For this review, take the finished solid that the model builds, in its own axes (mm). A direction names the side the tool comes from. Coordinates: 2 decimals unless noted, no trailing zeros. Write each loop counter-clockwise with the first axis right and the second up, starting at its lowest first coordinate (ties: lowest second). Pieces come first, ordered by that corner, then holes.
```python
from build123d import *

# Parameters (mm, degrees)
BOSS_EXTRUDE1_DEPTH = 370
SKETCH2_R           = 4.05
CUT_EXTRUDE1_DEPTH  = 26
CUT_EXTRUDE2_REACH  = 27
CUT_EXTRUDE3_REACH  = 27
SKETCH4_R           = 6


with BuildPart() as part:
    # Sketch1 → Boss-Extrude1 (new body)
    with BuildSketch(Plane.XY):
        with BuildLine():
            Line((2, 0), (23, 0))
            ThreePointArc((23, 0), (24.414213562, 0.585786438), (25, 2))
            Line((25, 2), (25, 23))
            ThreePointArc((25, 23), (24.414213562, 24.414213562), (23, 25))
            Line((23, 25), (2, 25))
            ThreePointArc((2, 25), (0.585786438, 24.414213562), (0, 23))
            Line((0, 23), (0, 2))
            ThreePointArc((0, 2), (0.585786438, 0.585786438), (2, 0))
        make_face()
        with BuildLine():
            Line((2, 1.25), (23, 1.25))
            ThreePointArc((23, 1.25), (23.530330086, 1.469669914), (23.75, 2))
            Line((23.75, 2), (23.75, 23))
            ThreePointArc((23.75, 23), (23.530330086, 23.530330086), (23, 23.75))
            Line((23, 23.75), (2, 23.75))
            ThreePointArc((2, 23.75), (1.469669914, 23.530330086), (1.25, 23))
            Line((1.25, 23), (1.25, 2))
            ThreePointArc((1.25, 2), (1.469669914, 1.469669914), (2, 1.25))
        make_face(mode=Mode.SUBTRACT)
    extrude(amount=BOSS_EXTRUDE1_DEPTH)

    # Sketch2 → Cut-Extrude1 (cut, through all)
    with BuildSketch(Plane(origin=(0, 25, 0), x_dir=(1, 0, 0), z_dir=(0, 1, 0))):
        with Locations((12.5, -293)):
            Circle(SKETCH2_R)
        with BuildLine():
            Line((8.45, -353), (8.45, -370))
            Line((8.45, -370), (16.55, -370))
            Line((16.55, -370), (16.55, -353))
            ThreePointArc((16.55, -353), (12.5, -348.95), (8.45, -353))
        make_face()
    extrude(amount=-CUT_EXTRUDE1_DEPTH, mode=Mode.SUBTRACT)

    # Sketch3 → Cut-Extrude2 (cut, up to next)
    with BuildSketch(Plane(origin=(0, 25, 0), x_dir=(1, 0, 0), z_dir=(0, 1, 0)), mode=Mode.PRIVATE) as cut_extrude2_sk1:
        with BuildLine():
            Line((17.05, -38), (17.05, -70))
            ThreePointArc((17.05, -70), (12.5, -74.55), (7.95, -70))
            Line((7.95, -70), (7.95, -38))
            ThreePointArc((7.95, -38), (12.5, -33.45), (17.05, -38))
        make_face()
    cut_extrude2_tool1 = extrude(cut_extrude2_sk1.sketch, amount=-CUT_EXTRUDE2_REACH, mode=Mode.PRIVATE) & part.part
    add(cut_extrude2_tool1.solids().sort_by_distance((12.5, 25, 54))[0], mode=Mode.SUBTRACT)

    # Sketch4 → Cut-Extrude3 (cut, up to next)
    with BuildSketch(Plane.XZ, mode=Mode.PRIVATE) as cut_extrude3_sk1:
        with Locations((12.5, 53)):
            Circle(SKETCH4_R)
    cut_extrude3_tool1 = extrude(cut_extrude3_sk1.sketch, amount=-CUT_EXTRUDE3_REACH, mode=Mode.PRIVATE) & part.part
    add(cut_extrude3_tool1.solids().sort_by_distance((12.5, 0, 53))[0], mode=Mode.SUBTRACT)
    # Sketch4 → Cut-Extrude3 (cut, up to next)
    with BuildSketch(Plane.XZ, mode=Mode.PRIVATE) as cut_extrude3_sk2:
        with BuildLine():
            Line((7.95, 0), (7.95, 17))
            ThreePointArc((7.95, 17), (12.5, 21.55), (17.05, 17))
            Line((17.05, 17), (17.05, 0))
            Line((17.05, 0), (7.95, 0))
        make_face()
    cut_extrude3_tool2 = extrude(cut_extrude3_sk2.sketch, amount=-CUT_EXTRUDE3_REACH, mode=Mode.PRIVATE) & part.part
    add(cut_extrude3_tool2.solids().sort_by_distance((12.5, 0, 10.311845))[0], mode=Mode.SUBTRACT)


solid = part.part
```
Q1. Add section D-D (z = 293). State the section outline as (x, y) points, then the cut area to 3 significant figures.
Ans:
outline: (0, 2) arc R2 ccw to (2, 0) - (8.45, 0) - (8.45, 1.25) - (2, 1.25) arc R0.75 cw to (1.25, 2) - (1.25, 23) arc R0.75 cw to (2, 23.75) - (8.45, 23.75) - (8.45, 25) - (2, 25) arc R2 ccw to (0, 23) - close; (16.55, 0) - (23, 0) arc R2 ccw to (25, 2) - (25, 23) arc R2 ccw to (23, 25) - (16.55, 25) - (16.55, 23.75) - (23, 23.75) arc R0.75 cw to (23.75, 23) - (23.75, 2) arc R0.75 cw to (23, 1.25) - (16.55, 1.25) - close
area: 95.5 mm2
Q2. Add section C-C (x = 12.5). State the section outline as (y, z) points, then the cut area to 3 significant figures.
Ans:
outline: (0, 21.55) - (1.25, 21.55) - (1.25, 47) - (0, 47) - close; (0, 59) - (1.25, 59) - (1.25, 288.95) - (0, 288.95) - close; (0, 297.05) - (1.25, 297.05) - (1.25, 348.95) - (0, 348.95) - close; (23.75, 0) - (25, 0) - (25, 33.45) - (23.75, 33.45) - close; (23.75, 74.55) - (25, 74.55) - (25, 288.95) - (23.75, 288.95) - close; (23.75, 297.05) - (25, 297.05) - (25, 348.95) - (23.75, 348.95) - close
area: 759 mm2
Q3. Clearance check with flat-ended pins moving along their axes: pin 1 Ø0.6 at (y, z) = (1, 361.5) entering from -X; pin 2 Ø1.4 at (y, z) = (24, 50) entering from +X; pin 3 Ø1.4 at (y, z) = (0.5, 7) entering from -X; pin 4 Ø8 at (x, y) = (15, 19) entering from -Z. State where each tip first meets the part, or that it passes through.
Ans:
pin 1: stops at x = 0.13
pin 2: stops at x = 24.98
pin 3: stops at x = 0.17
pin 4: passes through
Q4. Tool access review of faces 1 (the flat face through (24, 13, 370)), 2 (the cylindrical face through (18.04, 0.62, 50.7)), 3 (the flat face through (23.75, 12, 182)): name each direction out of +Z, -Z, +X, -X, +Y, -Y from which nothing blocks a thin tool from reaching the whole face with its end or side.
Ans:
face 1: +Z, +X, -X, +Y, -Y
face 2: -Y
face 3: +Z, -Z
Q5. Add section A-A (y = 11.25). State the section outline as (x, z) points.
Ans:
outline: (0, 0) - (1.25, 0) - (1.25, 370) - (0, 370) - close; (23.75, 0) - (25, 0) - (25, 370) - (23.75, 370) - close
Q6. For probe 1 along Z at (x, y) = (12.5, 24.15); probe 2 along Z at (x, y) = (12.5, 0.5); probe 3 along Y at (x, z) = (19.5, 221.5), list the stretches that pass through material, from the lowest coordinate up.
Ans:
probe 1: z = 0 to 33.45, 74.55 to 288.95, 297.05 to 348.95
probe 2: z = 21.55 to 47, 59 to 288.95, 297.05 to 348.95
probe 3: y = 0 to 1.25, 23.75 to 25
Q7. Draft analysis for pull direction Y (two halves, no side actions). For faces 4 (the flat face through (12, 1.25, 182)), 5 (the flat face through (25, 12, 182)), 6 (the flat face through (1.25, 13, 182)), 7 (the flat face through (13, 25, 182)), state which applies: +Y half, -Y half, draft (parallel to the pull), parting line (faces both ways), or undercut.
Ans:
face 4: undercut
face 5: draft
face 6: undercut
face 7: +Y half
Q8. Add section B-B (z = 199.5). State the section outline as (x, y) points, then the cut area to 3 significant figures.
Ans:
outline: (0, 2) arc R2 ccw to (2, 0) - (23, 0) arc R2 ccw to (25, 2) - (25, 23) arc R2 ccw to (23, 25) - (2, 25) arc R2 ccw to (0, 23) - close; hole (1.25, 2) arc R0.75 ccw to (2, 1.25) - (23, 1.25) arc R0.75 ccw to (23.75, 2) - (23.75, 23) arc R0.75 ccw to (23, 23.75) - (2, 23.75) arc R0.75 ccw to (1.25, 23) - close
area: 116 mm2
